Geometry check sheet. Reference: drawing and pictorial views, mm from the part's lowest x, y, z. A direction names the side the tool comes from. Round coordinates to 2 decimals unless told otherwise and drop trailing zeros. Loops run counter-clockwise (first coordinate to the right, second up) from the corner with the lowest first, then second, coordinate; pieces in that order, holes last. Notation, with made-up numbers: (34, 36) - (60, 36) arc R10 ccw to (60, 50) - close; hole circle Ø6 at (48.25, 28). An arc over 180 degrees is marked (long way). Return JSON: item names as keys, results as strings.
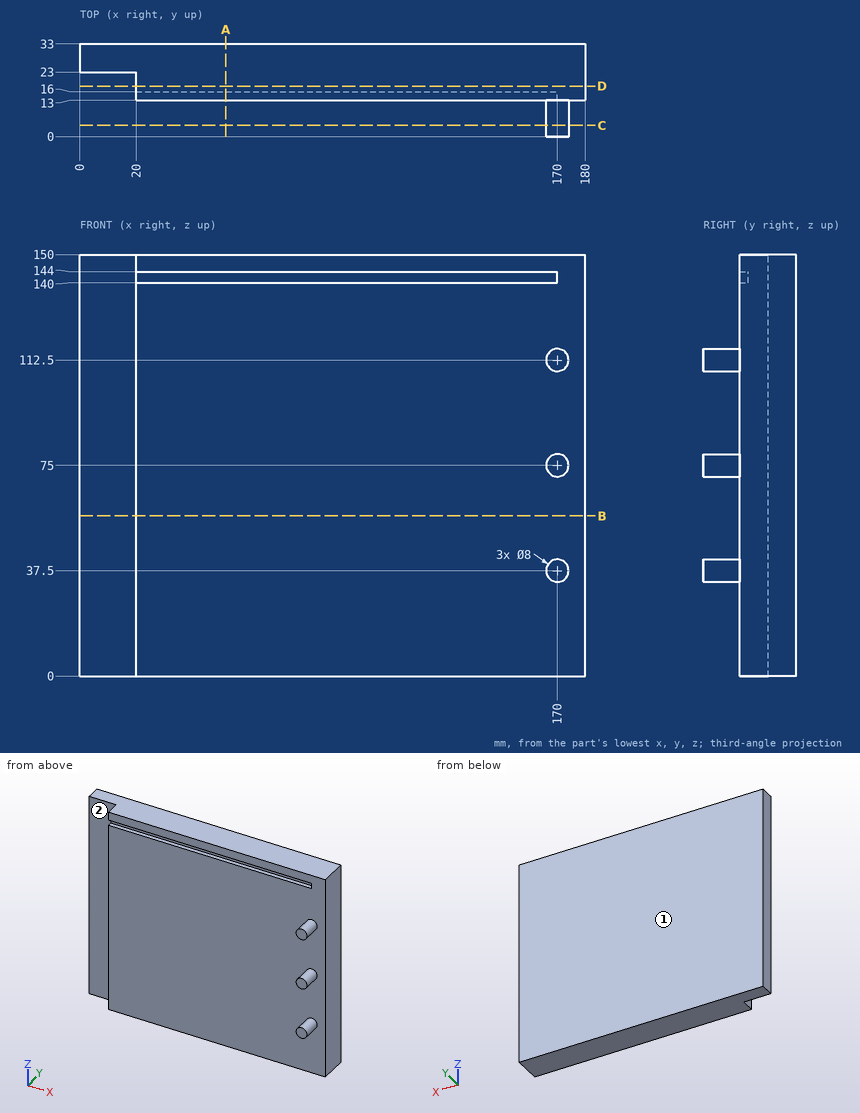
Q1. Depth check by flat-ended pin: P1, Ø10, axis at y = 11, z = 45, coming from the +X side; P2, Ø16, axis at x = 10, z = 75, coming from the -Y side; P3, Ø0.9, axis at y = 14, z = 141.5, coming from the -X side; P4, Ø4, axis at x = 156.5, z = 58, coming from the -Y side. Enter the tip coordinate at first touch or a pass-through.
Answer key:
{"P1": "stops at x = 180", "P2": "stops at y = 23", "P3": "stops at x = 170", "P4": "stops at y = 13"}
Q2. Sectioned sample at D-D (y = 18). Enter the section's corners in (x, z).
Answer key:
{"outline": "(20, 0) - (180, 0) - (180, 150) - (20, 150) - close"}
Q3. Sectioned sample at A-A (x = 52). Enter the section's corners in (y, z).
Answer key:
{"outline": "(13, 0) - (33, 0) - (33, 150) - (13, 150) - (13, 144) - (16, 144) - (16, 140) - (13, 140) - close"}
Q4. Scan lines: probe 1 along Y at (x, z) = (157.5, 107.5); probe 2 along X at (y, z) = (18, 77). Record each from-to range of solid material in increasing order. Write a range as [from, to].
Answer key:
{"probe 1": "y = [13, 33]", "probe 2": "x = [20, 180]"}
Q5. Sectioned sample at C-C (y = 4). Enter the section's corners in (x, z), plus the area to 3 significant figures.
Answer key:
{"outline": "circle Ø8 at (170, 37.5); circle Ø8 at (170, 75); circle Ø8 at (170, 112.5)", "area": "151 mm²"}
Q6. Tool access check on the marked faces 1 and 2. Record the directions out of +Z, -Z, +X, -X, +Y, -Y that give a thin tool (end or side, any length) a straight path to the whole face; none if there is none.
Answer key:
{"face 1": "+Z, -Z, +X, -X, +Y", "face 2": "+Z, -Z, -X, -Y"}
Q7. Sectioned sample at B-B (z = 57). Enter the section's corners in (x, y), plus the area to 3 significant figures.
Answer key:
{"outline": "(0, 23) - (20, 23) - (20, 13) - (180, 13) - (180, 33) - (0, 33) - close", "area": "3,400 mm²"}
